Verification items for the finished model (mm, model axes). Face numbers are marked on the shaded views. Coordinates: 2 decimals unless noted, no trailing zeros. Order: outer loops, then holes, each group sorted by start corner. A loop starts at its lowest first (then second) coordinate and runs counter-clockwise, first axis right, second up. Notation, with made-up numbers: M 86,47 L 130,47 A9 ccw 130,59 Z; hole C 67,-31.5 d5. An arc over 180 degrees is marked long. Return JSON: item names as keys, results as strings. Group by question number.
Q1. Section check C-C, the plane y = 13.5. Enter the section's corners in (x, z), then the cut area to 3 significant figures.
Q2. Section check A-A, the plane z = 6. Enter the section's corners in (x, y), then the cut area to 3 significant figures.
Q3. Section check B-B, the plane x = -5.75. Enter the section's corners in (y, z).
Q4. Thickness scan on probe 1 along Z at (x, y) = (-7.75, 4); probe 2 along X at (y, z) = (67, 16.25); probe 3 along Z at (x, y) = (-3.75, 21). Record the ranges inside material, lowest first.
Q5. Mould release check, pull along Z, two halves, no side actions. Record for the marked faces 1, 2, 3 and 4: pulls with the +Z half, pulls with the -Z half, needs draft (parallel to the pull), parting line crosses it, or undercut.
Q6. Section check D-D, the plane y = 29. Enter the section's corners in (x, z), then the cut area to 3 significant figures.
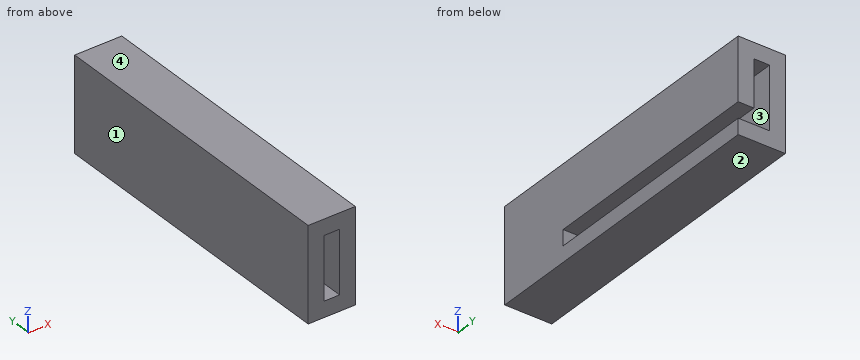
from build123d import *

# Parameters (mm, degrees)
F0_W     = 12
F0_H     = 80
F1_DEPTH = 24
F2_W     = 4
F2_H     = 16
F3_DEPTH = 9900
F4_W     = 60
F4_H     = 4
F5_DEPTH = 4


with BuildPart() as f1:
    # F0 (on Top) → F1 (new body)
    with BuildSketch(Plane.XY):
        with Locations((-6, 40)):
            Rectangle(F0_W, F0_H)
    extrude(amount=F1_DEPTH)

    # F2 (on face) → F3 (cut)
    with BuildSketch(Plane.XZ):
        with Locations((-6, 12)):
            Rectangle(F2_W, F2_H)
    extrude(amount=-F3_DEPTH, mode=Mode.SUBTRACT)

    # F4 (on face) → F5 (cut)
    with BuildSketch(Plane.YZ):
        with Locations((50, 6)):
            Rectangle(F4_W, F4_H)
    extrude(amount=-F5_DEPTH, mode=Mode.SUBTRACT)


solid = f1.part
Numbers:
{
 "1": {"outline": "M -12,0 L 0,0 L 0,24 L -12,24 Z; hole M -8,4 L -4,4 L -4,20 L -8,20 Z", "area": "224 mm2"},
 "2": {"outline": "M -12,0 L -8,0 L -8,80 L -12,80 Z; M -4,0 L 0,0 L 0,20 L -4,20 Z", "area": "400 mm2"},
 "3": {"outline": "M 0,0 L 80,0 L 80,4 L 0,4 Z; M 0,20 L 80,20 L 80,24 L 0,24 Z"},
 "4": {"probe 1": "z = 0 to 4, 20 to 24", "probe 2": "x = -12 to -8, -4 to 0", "probe 3": "z = 0 to 4, 8 to 24"},
 "5": {"face 1": "needs draft", "face 2": "pulls with the -Z half", "face 3": "undercut", "face 4": "pulls with the +Z half"},
 "6": {"outline": "M -12,0 L 0,0 L 0,4 L -8,4 L -8,20 L -4,20 L -4,8 L 0,8 L 0,24 L -12,24 Z", "area": "208 mm2"}
}
